Work out the finished part from the listing and answer in its coordinate system (mm). Face numbers are marked on the shaded views. A direction names the side the tool comes from. Give positions to 0.01 mm unless a question says otherwise; leave off trailing zeros. Loops run counter-clockwise (first coordinate to the right, second up) from the corner with the lowest first, then second, coordinate; pieces in that order, holes last. Notation, with made-up numbers: M 31,22.5 L 87,22.5 A24 cw 87,44.5 Z; hole C -19,19.5 d11. An arc over 180 degrees is marked long. Answer as a JSON object with one key per item and string values. Group by question number.
```python
from build123d import *

# Parameters (mm, degrees)
F1_DEPTH    = 25
F2_W        = 6
F2_H        = 13
F3_DEPTH    = 12.5
F4_SIZE2    = 1
F4_SIZE     = 1
F5_T1_DEPTH = 25
F5_T3_DEPTH = 35


# Not quite as in the source:
# - a fillet or chamfer that OpenCascade refuses, or shapes differently, is made with other operations: its cross-section is extruded or revolved along the edge and cut away or added


with BuildPart() as f1:
    # F0 (on Top) → F1 (new body)
    with BuildSketch(Plane.XY):
        Polygon((-55.1361331344, -5), (-52.1361331344, -5), (-52.1361331344, 35), (19.8638668656, 35), (19.8638668656, -10), (19.8638668656, -13), (30.8638668656, -13), (33.8638668656, -13), (33.8638668656, -10), (33.8638668656, 0), (30.8638668656, 0), (30.8638668656, -10), (22.8638668656, -10), (22.8638668656, 38), (-55.1361331344, 38), align=None)
    extrude(amount=F1_DEPTH)

    # F2 (on face) → F3 (cut, symmetric)
    with BuildSketch(Plane(origin=(-55.1361331344, 0, 0), x_dir=(0, -1, 0), z_dir=(-1, 0, 0))):
        with Locations((-12, 12.5)):
            Rectangle(F2_W, F2_H)
    extrude(amount=F3_DEPTH, both=True, mode=Mode.SUBTRACT)

    # F4
    f4_edges = [f1.edges().sort_by_distance(p)[0] for p in [
        (-55.136133, 12, 19),
        (-55.136133, 15, 12.5),
        (-55.136133, 9, 12.5),
        (-55.136133, 12, 6),
    ]]
    chamfer(f4_edges, length=F4_SIZE, length2=F4_SIZE2)

    # F5: fillet of radius 2 on 10 edges, made by hand

    # F5_s2 → F5_t1 (join)
    with BuildSketch(Plane.XY):
        with BuildLine():
            ThreePointArc((22.8638668656, -8), (23.4496533033, -9.4142135624), (24.8638668656, -10))
            Line((24.8638668656, -10), (22.8638668656, -10))
            Line((22.8638668656, -10), (22.8638668656, -8))
        make_face()
        with BuildLine():
            ThreePointArc((30.8638668656, -8), (30.278080428, -9.4142135624), (28.8638668656, -10))
            Line((28.8638668656, -10), (30.8638668656, -10))
            Line((30.8638668656, -10), (30.8638668656, -8))
        make_face()
    extrude(amount=F5_T1_DEPTH)

    # F5_s4 → F5_t3 (cut)
    with BuildSketch(Plane.XY.offset(-5)):
        with BuildLine():
            ThreePointArc((-55.1361331344, 36), (-54.5503466967, 37.4142135624), (-53.1361331344, 38))
            Line((-53.1361331344, 38), (-55.1361331344, 38))
            Line((-55.1361331344, 38), (-55.1361331344, 36))
        make_face()
        with BuildLine():
            ThreePointArc((20.8638668656, 38), (22.278080428, 37.4142135624), (22.8638668656, 36))
            Line((22.8638668656, 36), (22.8638668656, 38))
            Line((22.8638668656, 38), (20.8638668656, 38))
        make_face()
        with BuildLine():
            ThreePointArc((19.8638668656, -11), (20.4496533033, -12.4142135624), (21.8638668656, -13))
            Line((21.8638668656, -13), (19.8638668656, -13))
            Line((19.8638668656, -13), (19.8638668656, -11))
        make_face()
        with BuildLine():
            ThreePointArc((31.8638668656, -13), (33.278080428, -12.4142135624), (33.8638668656, -11))
            Line((33.8638668656, -11), (33.8638668656, -13))
            Line((33.8638668656, -13), (31.8638668656, -13))
        make_face()
        with BuildLine():
            ThreePointArc((33.8638668656, -2), (33.278080428, -0.5857864376), (31.8638668656, 0))
            Line((31.8638668656, 0), (33.8638668656, 0))
            Line((33.8638668656, 0), (33.8638668656, -2))
        make_face()
        with BuildLine():
            ThreePointArc((32.8638668656, 0), (31.4496533033, -0.5857864376), (30.8638668656, -2))
            Line((30.8638668656, -2), (30.8638668656, 0))
            Line((30.8638668656, 0), (32.8638668656, 0))
        make_face()
        with BuildLine():
            ThreePointArc((-55.1361331344, -3), (-54.5503466967, -4.4142135624), (-53.1361331344, -5))
            Line((-53.1361331344, -5), (-55.1361331344, -5))
            Line((-55.1361331344, -5), (-55.1361331344, -3))
        make_face()
        with BuildLine():
            ThreePointArc((-54.1361331344, -5), (-52.721919572, -4.4142135624), (-52.1361331344, -3))
            Line((-52.1361331344, -3), (-52.1361331344, -5))
            Line((-52.1361331344, -5), (-54.1361331344, -5))
        make_face()
    extrude(amount=F5_T3_DEPTH, mode=Mode.SUBTRACT)


solid = f1.part
```
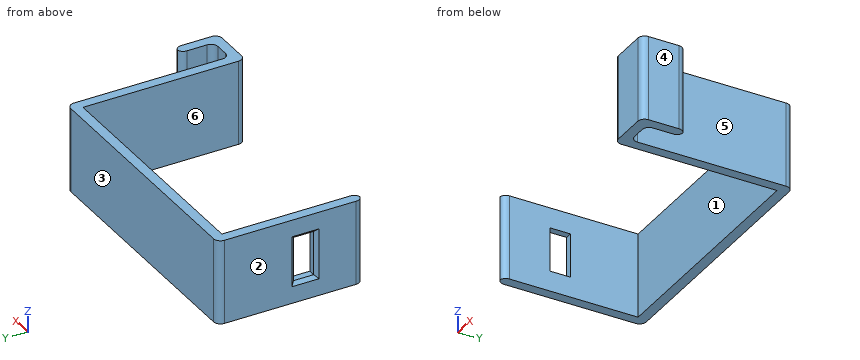
Item 1: A cutting plane is placed at D-D (z = 21). Determine the outline of the cut face in (x, y), and give its area (3 significant figures).
Item 2: A cutting plane is placed at B-B (y = -6.5). Determine the outline of the cut face in (x, z), and give its area (3 significant figures).
Item 3: A cutting plane is placed at A-A (y = 11). Determine the outline of the cut face in (x, z).
Item 4: For a pull along X with two mould halves and no side action, classify the marked faces 1, 2 and 3 as pulls with the +X half, pulls with the -X half, needs draft (parallel to the pull), parting line crosses it, or undercut.
Item 5: Find the intervals of material crossed by probe 1 along X at (y, z) = (3, 21); probe 2 along Y at (x, z) = (18, 9); probe 3 along Y at (x, z) = (22, 8.25), in increasing order. Write a range as [from, to].
Item 6: A cutting plane is placed at C-C (z = 12). Determine the outline of the cut face in (x, y), and give its area (3 significant figures).
Item 7: Given pin 1 Ø1 at (x, z) = (-53, 15) entering from -Y; pin 2 Ø8 at (x, y) = (-18.5, 28.5) entering from +Z; pin 3 Ø1 at (x, z) = (1.5, 9.5) entering from -Y; pin 4 Ø7.5 at (y, z) = (10, 18) entering from +X, each flat-ended and moving along its own axis, determine where each tip first touches the part or whether it passes through.
Item 8: A tool of negligible diameter and unlimited length cuts with its end or side. For the marked faces 4, 5 and 6, from which of +Z, -Z, +X, -X, +Y, -Y can it reach the whole face along a straight path? Write none if from no direction.
The answers:
{
 "1": {"outline": "M -55.14,-3 A2 ccw -53.64,-4.94 A2 ccw -52.14,-3 L -52.14,35 L 19.86,35 L 19.86,-11 A2 ccw 21.86,-13 L 31.86,-13 A2 ccw 33.86,-11 L 33.86,-2 A2 ccw 32.36,-0.06 A2 ccw 30.86,-2 L 30.86,-8 A2 cw 28.86,-10 L 24.86,-10 A2 cw 22.86,-8 L 22.86,36 A2 ccw 20.86,38 L -53.14,38 A2 ccw -55.14,36 Z", "area": "556 mm^2"},
 "2": {"outline": "M 19.86,0 L 22.86,0 L 22.86,25 L 19.86,25 Z; M 30.86,0 L 33.86,0 L 33.86,25 L 30.86,25 Z", "area": "150 mm^2"},
 "3": {"outline": "M -55.14,0 L -52.14,0 L -52.14,6 L -54.14,6 L -55.14,5 Z; M -55.14,20 L -54.14,19 L -52.14,19 L -52.14,25 L -55.14,25 Z; M 19.86,0 L 22.86,0 L 22.86,25 L 19.86,25 Z"},
 "4": {"face 1": "undercut", "face 2": "pulls with the -X half", "face 3": "needs draft"},
 "5": {"probe 1": "x = [-55.14, -52.14], [19.86, 22.86]", "probe 2": "y = [35, 38]", "probe 3": "y = [-13, 37.65]"},
 "6": {"outline": "M -55.14,-3 A2 ccw -53.64,-4.94 A2 ccw -52.14,-3 L -52.14,9 L -54.14,9 L -55.14,8 Z; M -55.14,16 L -54.14,15 L -52.14,15 L -52.14,35 L 19.86,35 L 19.86,-11 A2 ccw 21.86,-13 L 31.86,-13 A2 ccw 33.86,-11 L 33.86,-2 A2 ccw 32.36,-0.06 A2 ccw 30.86,-2 L 30.86,-8 A2 cw 28.86,-10 L 24.86,-10 A2 cw 22.86,-8 L 22.86,36 A2 ccw 20.86,38 L -53.14,38 A2 ccw -55.14,36 Z", "area": "537 mm^2"},
 "7": {"pin 1": "stops at y = -4.9", "pin 2": "passes through", "pin 3": "stops at y = 35", "pin 4": "stops at x = 22.86"},
 "8": {"face 4": "+Z, -Z, +X, +Y, -Y", "face 5": "+Z, -Z, +Y", "face 6": "+Z, -Z, -Y"}
}
